```python
from build123d import *

# Parameters (mm, degrees)
F4_DEPTH = 65.001
F5_T     = -1


with BuildPart() as f1:
    # F0 (on Front) → F1 (revolve)
    with BuildSketch(Plane.XZ):
        with BuildLine():
            Line((-15, 50), (-15, 0))
            ThreePointArc((-15, 0), (-10.606602, -10.606602), (0, -15))
            Line((0, -15), (0, 50))
            Line((0, 50), (-15, 50))
        make_face()
    revolve(axis=Axis((0, 0, 17.5), (0, 0, 1)))

    # F3 (on offset) → F4 (cut, through all)
    with BuildSketch(Plane.XY.offset(50)):
        with BuildLine():
            Line((-15, 0), (15, 0))
            ThreePointArc((15, 0), (0, 15), (-15, 0))
        make_face()
    extrude(amount=-F4_DEPTH, mode=Mode.SUBTRACT)

    # F5
    f5_openings = [f1.faces().sort_by_distance(p)[0] for p in [
        (0, 0, 19.018801),
        (0, -6.366198, 50),
    ]]
    offset(amount=F5_T, openings=f5_openings)


solid = f1.part
```
Geometry check sheet. Reference: the model listing, model coordinates, mm. Round coordinates to 2 decimals unless told otherwise and drop trailing zeros. Loops run counter-clockwise (first coordinate to the right, second up) from the corner with the lowest first, then second, coordinate; pieces in that order, holes last. Notation, with made-up numbers: M 87.25,-24.75 L 107.25,-24.75 A27 cw 107.25,-7.75 Z; hole C -35,54 d1. An arc over 180 degrees is marked long. Return JSON: item names as keys, results as strings. Group by question number.
(1) Section check A-A, the plane z = 38. Enter the section's corners in (x, y), and give its area (3 significant figures).
(2) Go/stop test with flat-tipped pins: pin 1 (8 mm diameter, centred on x = -7.5, z = 1, fed in from -Y); pin 2 (8 mm diameter, centred on x = -7, y = -5, fed in from +Z); pin 3 (6 mm diameter, centred on x = -10, y = -11, fed in from -Z). Record where each tip stops, or that it passes through.
(3) Scan lines: line 1 along X through (y, z) = (-8.5, 22.5); line 2 along X through (y, z) = (-5.75, -10); line 3 along Z through (x, y) = (-8.5, -7). Record each from-to range of solid material in increasing order. Write a range as [from, to].
(4) Mould release check, pull along X, two halves, no side actions. Record for faces 1 (the face through (0, -15, 25)), 2 (the face through (-0.1, -14.2, 50)), 3 (the face through (0, -14, 25)): pulls with the +X half, pulls with the -X half, needs draft (parallel to the pull), parting line crosses it, or undercut.
Data:
{
 "1": {"outline": "M -15,0 A15 ccw 15,0 L 14,0 A14 cw -14,0 Z", "area": "45.6 mm²"},
 "2": {"pin 1": "y = -14.59", "pin 2": "z = -6.1", "pin 3": "z = -9.18"},
 "3": {"line 1": "[-12.36, -11.12], [11.12, 12.36]", "line 2": "[-9.59, -7.93], [7.93, 9.59]", "line 3": "[-10.19, -8.65]"},
 "4": {"face 1": "parting line crosses it", "face 2": "needs draft", "face 3": "undercut"}
}
